```python
from build123d import *

# Parameters (mm, degrees)
F0_R     = 2.85
F0_R_2   = 1.5
F1_DEPTH = 3.22
F2_DEPTH = 8
F3_R     = 0.4
F4_R     = 0.2
F5_SIZE  = 0.2
F6_START = 1.32
F6_DEPTH = 23.68
F7_SIZE  = 0.1


# Not quite as in the source:
# - an extrude whose draft closes it to a point is written as a loft to that point


with BuildPart() as f1:
    # F0 (on Top) → F1 (new body)
    with BuildSketch(Plane.XY):
        Circle(F0_R)
        Circle(F0_R_2, mode=Mode.SUBTRACT)
        Circle(F0_R_2)
        Polygon((-1.3465408328, -0.0965804618), (-0.7569115498, 1.1178483376), (0.589629283, 1.2144287993), (1.3465408328, 0.0965804618), (0.7569115498, -1.1178483376), (-0.589629283, -1.2144287993), align=None, mode=Mode.SUBTRACT)
        Polygon((0.589629283, 1.2144287993), (-0.7569115498, 1.1178483376), (-1.3465408328, -0.0965804618), (-0.589629283, -1.2144287993), (0.7569115498, -1.1178483376), (1.3465408328, 0.0965804618), align=None)
    extrude(amount=F1_DEPTH)

    # F0 (on Top) → F2 (join)
    with BuildSketch(Plane.XY):
        Circle(F0_R_2)
        Polygon((-1.3465408328, -0.0965804618), (-0.7569115498, 1.1178483376), (0.589629283, 1.2144287993), (1.3465408328, 0.0965804618), (0.7569115498, -1.1178483376), (-0.589629283, -1.2144287993), align=None, mode=Mode.SUBTRACT)
        Polygon((0.589629283, 1.2144287993), (-0.7569115498, 1.1178483376), (-1.3465408328, -0.0965804618), (-0.589629283, -1.2144287993), (0.7569115498, -1.1178483376), (1.3465408328, 0.0965804618), align=None)
    extrude(amount=-F2_DEPTH)

    # F3
    f3_edges = [f1.edges().sort_by_distance(p)[0] for p in [
        (-2.85, 0, 3.22),
    ]]
    fillet(f3_edges, radius=F3_R)

    # F4
    f4_edges = [f1.edges().sort_by_distance(p)[0] for p in [
        (-2.85, 0, 0),
    ]]
    fillet(f4_edges, radius=F4_R)

    # F5
    f5_edges = [f1.edges().sort_by_distance(p)[0] for p in [
        (-1.5, 0, -8),
    ]]
    chamfer(f5_edges, length=F5_SIZE)

    # F0 (on Top) → F6 (cut)
    with BuildSketch(Plane.XY.offset(F6_START)):
        Polygon((0.589629283, 1.2144287993), (-0.7569115498, 1.1178483376), (-1.3465408328, -0.0965804618), (-0.589629283, -1.2144287993), (0.7569115498, -1.1178483376), (1.3465408328, 0.0965804618), align=None)
    extrude(amount=F6_DEPTH, mode=Mode.SUBTRACT)

    # F7
    f7_edges = [f1.edges().sort_by_distance(p)[0] for p in [
        (-1.051726, 0.510634, 3.22),
        (-0.083641, 1.166139, 3.22),
        (0.968085, 0.655505, 3.22),
        (1.051726, -0.510634, 3.22),
        (0.083641, -1.166139, 3.22),
        (-0.968085, -0.655505, 3.22),
    ]]
    chamfer(f7_edges, length=F7_SIZE)

    # F6_face (on face) → F8 section 0
    with BuildSketch(Plane.XY.offset(1.32), mode=Mode.PRIVATE) as f8_s0:
        Polygon((1.3465408328, 0.0965804618), (0.589629283, 1.2144287993), (-0.7569115498, 1.1178483376), (-1.3465408328, -0.0965804618), (-0.589629283, -1.2144287993), (0.7569115498, -1.1178483376), align=None)
    loft([f8_s0.sketch, Vertex(0, 0, 1.217714003)], ruled=True, mode=Mode.SUBTRACT)


solid = f1.part
```
Geometry check sheet. Reference: the model listing, model coordinates, mm. A direction names the side the tool comes from. Coordinates: 2 decimals unless noted, no trailing zeros. Order: outer loops, then holes, each group sorted by start corner. A loop starts at its lowest first (then second) coordinate and runs counter-clockwise, first axis right, second up. Notation, with made-up numbers: (-27, 75.25) - (-1, 75.25) arc R19 ccw to (-1, 84.25) - close; hole circle Ø10 at (-25, 17.25). An arc over 180 degrees is marked (long way). Use one line per item in the form item = value.
1. Scan lines: line 1 (Z direction, x = 0.2, y = 1.65); line 2 (X direction, y = 0.2, z = 2.75); line 3 (X direction, y = 1.45, z = 2.5). Record each from-to range of solid material in increasing order.
Here are the results:
line_1 = 0 to 3.22
line_2 = -2.84 to -1.2, 1.28 to 2.84
line_3 = -2.45 to 2.45
2. Draft check along Y on faces 1 (the face through (2, 0, 0)), 2 (the face through (-0.074, 1.167, 2.207)), 3 (the face through (0.63, -0.32, 1.28)), 4 (the face through (-2.262, -1.734, 1.492)). Enter one of: pulls with the +Y half, pulls with the -Y half, needs draft (parallel to the pull), parting line crosses it, or undercut.
Here are the results:
face_1 = needs draft
face_2 = undercut
face_3 = undercut
face_4 = parting line crosses it
3. Section check A-A (z = -4). Record the boundary of the cut face in (x, y).
Here are the results:
outline = circle Ø3 at (0, 0)
4. Gauge pin test, flat ends, axial feed: pin 1 (3 mm diameter, centred on x = 1.5, z = -2, fed in from -Y); pin 2 (2 mm diameter, centred on x = -1.5, z = -5.5, fed in from -Y); pin 3 (1.5 mm diameter, centred on y = -0.5, z = -0.5, fed in from -X). Record the tip position at first contact, or that the pin passes through.
Here are the results:
pin_1 = -1.5
pin_2 = -1.41
pin_3 = -2.84
5. Access from +Z, -Z, +X, -X, +Y, -Y to the whole of each face (thin tool, end or side, straight path). Record for faces 5 (the face through (0, 0, -8)), 6 (the face through (-1.5, 0.07, -3.85)), 7 (the face through (0.59, 0.39, 1.28)).
Here are the results:
face_5 = -Z, +X, -X, +Y, -Y
face_6 = -Z
face_7 = +Z
